Could you check a few things on this model? Use its own coordinates, in mm. A direction names the side the tool comes from. Give positions to 0.01 mm unless a question says otherwise; leave off trailing zeros. Order: outer loops, then holes, each group sorted by start corner. A loop starts at its lowest first (then second) coordinate and runs counter-clockwise, first axis right, second up.
(1) Imagine slicing it at D-D, the plane z = 1.75. Write out the boundary of the cut face in (x, y).
(2) On a 3-axis mill with a long thin cutter (end or side, diameter ignored), from which of +Z, -Z, +X, -X, +Y, -Y can I reach the whole of each face in a straight line? I mean faces 1 (the flat face through (-1, 2, 8.75)), 2 (the cylindrical face through (-6.944, -5.324, 1.232)). Say none if no direction works.
(3) Will these pins go through, and if not, where does the flat tip stop? pin 1 (1.5 mm diameter, centred on x = 2.5, z = 4, fed in from -Y); pin 2 (3 mm diameter, centred on x = -6.5, z = 2.5, fed in from -Y); pin 3 (8 mm diameter, centred on x = 6, y = -1.5, fed in from +Z).
(4) If we mould it in two halves opening along Z, with no side actions, what happens to faces 3 (the flat face through (0, 0, 9.75)), 4 (the flat face through (0, 0, 0)), 5 (the cylindrical face through (0, -2, 6))? For each: released by +Z, released by -Z, zero draft, split by the parting line, or undercut.
(5) Imagine slicing it at A-A, the plane x = 0. Write out the boundary of the cut face in (y, z), then the cut area to 4 significant figures.
(6) If I drill on probe 1 along Z at (x, y) = (-6, -4.75); probe 2 along Z at (x, y) = (-2, -0.5); probe 3 along Y at (x, z) = (-1, 3.75), over which ranges is the centre line in solid material (lowest first)?
(7) Imagine slicing it at C-C, the plane y = -7. Write out the boundary of the cut face in (x, z).
(8) Imagine slicing it at B-B, the plane z = 6. Write out the boundary of the cut face in (x, y), then the cut area to 3 significant figures.
from build123d import *

# Parameters (mm, degrees)
F0_R     = 8.75
F1_DEPTH = 2.5
F2_R     = 2
F3_DEPTH = 6.25
F4_R     = 2.5
F6_R     = 2


with BuildPart() as f1:
    # F0 (on Top) → F1 (new body)
    with BuildSketch(Plane.XY):
        Circle(F0_R)
    extrude(amount=F1_DEPTH)

    # F2 (on face) → F3 (join)
    with BuildSketch(Plane.XY.offset(2.5)):
        Circle(F2_R)
    extrude(amount=F3_DEPTH)

    # F4 (on face) → F7 section 0
    with BuildSketch(Plane.XY.offset(8.75)):
        Circle(F4_R)
    # F6 (on offset) → F7 section 1
    with BuildSketch(Plane.XY.offset(9.75)):
        Circle(F6_R)
    loft()


solid = f1.part
Answer block:
1. outline: circle Ø17.5 at (0, 0)
2. face 1: none
2. face 2: +Z, -Z
3. pin 1: stops at y = -0.97
3. pin 2: stops at y = -7.18
3. pin 3: stops at z = 9.38
4. face 3: released by +Z
4. face 4: released by -Z
4. face 5: undercut
5. outline: (-8.75, 0) - (8.75, 0) - (8.75, 2.5) - (2, 2.5) - (2, 8.75) - (2.5, 8.75) - (2, 9.75) - (-2, 9.75) - (-2.5, 8.75) - (-2, 8.75) - (-2, 2.5) - (-8.75, 2.5) - close
5. area: 73.25 mm2
6. probe 1: z = 0 to 2.5
6. probe 2: z = 0 to 2.5, 8.75 to 9.63
6. probe 3: y = -1.73 to 1.73
7. outline: (-5.25, 0) - (5.25, 0) - (5.25, 2.5) - (-5.25, 2.5) - close
8. outline: circle Ø4 at (0, 0)
8. area: 12.6 mm2
